Design review of the part built by this model. Coordinates are the model's own, in mm. Face numbers are marked on the shaded views. A direction names the side the tool comes from. Round coordinates to 2 decimals unless told otherwise and drop trailing zeros. Write each loop counter-clockwise with the first axis right and the second up, starting at its lowest first coordinate (ties: lowest second). Pieces come first, ordered by that corner, then holes. Notation, with made-up numbers: (-3, 59.5) - (42, 59.5) arc R10 ccw to (42, 75.5) - close; hole circle Ø8 at (-31.5, -20). An arc over 180 degrees is marked (long way). Use one line per item in the form item = value.
```python
from build123d import *

# Parameters (mm, degrees)
F1_DEPTH = 61.087


with BuildPart() as f1:
    # F0 (on Front) → F1 (new body)
    with BuildSketch(Plane.XZ):
        Polygon((-14.4272, 37.735204), (-16.0782, 37.735204), (-16.0782, 13.732204), (42.0878, 13.732204), (42.0878, 37.735204), (40.4368, 37.735204), (40.4368, 17.034204), (33.6804, 17.034204), (33.6804, 37.735204), (32.0294, 37.735204), (32.0294, 17.034204), (28.067, 17.034204), (28.067, 37.735204), (26.416, 37.735204), (26.416, 17.034204), (22.4536, 17.034204), (22.4536, 37.735204), (20.8026, 37.735204), (20.8026, 17.034204), (16.8402, 17.034204), (16.8402, 37.735204), (15.1892, 37.735204), (15.1892, 17.034204), (11.2268, 17.034204), (11.2268, 37.735204), (9.5758, 37.735204), (9.5758, 17.034204), (5.6134, 17.034204), (5.6134, 37.735204), (3.9624, 37.735204), (3.9624, 17.034204), (0, 17.034204), (0, 37.735204), (-1.651, 37.735204), (-1.651, 17.034204), (-5.6134, 17.034204), (-5.6134, 37.735204), (-7.2644, 37.735204), (-7.2644, 17.034204), (-14.4272, 17.034204), align=None)
    extrude(amount=F1_DEPTH)


solid = f1.part
```
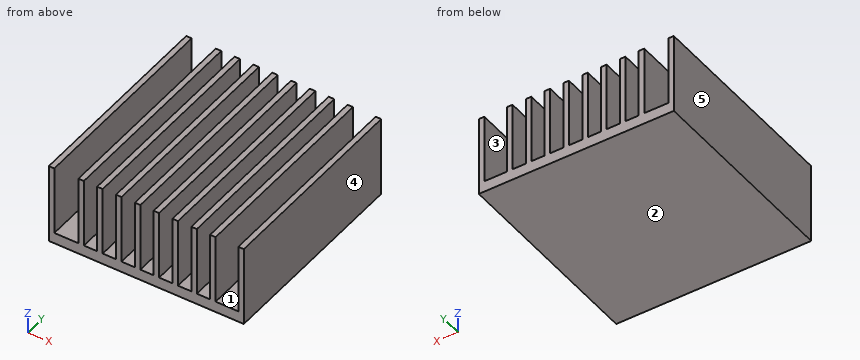
Q1. Draft analysis for pull direction X (two halves, no side actions). For the marked faces 3, 4 and 5, state which applies: released by +X, released by -X, zero draft, split by the parting line, or undercut.
Calculated:
face_3 = undercut
face_4 = released by +X
face_5 = released by -X
Q2. For P1, Ø4.5, axis at x = 24, y = -32, coming from the +Z side; P2, Ø1, axis at x = 36, y = -49, coming from the +Z side, all flat-tipped, find the tip position at first contact; note any pin that passes through.
Calculated:
P1 = 37.74
P2 = 17.03
Q3. Machinability: for the marked faces 1 and 2, which of the approach directions +Z, -Z, +X, -X, +Y, -Y give a long, thin tool a straight path to every point of the face, cutting with its end or side? Answer none if there is none.
Calculated:
face_1 = +Z, +Y, -Y
face_2 = -Z, +X, -X, +Y, -Y
Q4. We need section B-B on x = 7. Write out the cut boundary in (y, z), then the cut area to 3 significant figures.
Calculated:
outline = (-61.09, 13.73) - (0, 13.73) - (0, 17.03) - (-61.09, 17.03) - close
area = 202 mm2
Q5. We need section A-A on z = 35.75. State how many separate pieces and enclosed holes the cut face has, then the cut area to 3 significant figures.
Calculated:
separate_pieces = 10
enclosed_holes = 0
area = 1,010 mm2
Q6. To check wall thickness, follow line 1 along Z through (x, y) = (-10, -52). State the ranges of the line that lie inside material, in increasing order. Write a range as from..to.
Calculated:
line_1 = 13.73..17.03
